Source: three-view drawing plus pictorial views. Frame: mm from the lowest corner of the part. Give positions to 0.01 mm unless a question says otherwise; leave off trailing zeros. Write each loop counter-clockwise with the first axis right and the second up, starting at its lowest first coordinate (ties: lowest second). Pieces come first, ordered by that corner, then holes.
Q1. Pin query (flat end, axial travel): pin 1 (9.5 mm diameter, centred on x = 13, z = 256, fed in from -Y); pin 2 (3 mm diameter, centred on x = 7, y = 86.5, fed in from +Z); pin 3 (3 mm diameter, centred on x = 12.5, y = 304.5, fed in from +Z). Return the tip coordinate at first contact, or that it passes through.
Q2. Cut plane B-B on x = 7.75. Return the cut outline in (y, z).
Q3. Draft query along X for the marked faces 1 and 2. Return one class per face: pulls with the +X half, pulls with the -X half, needs draft (parallel to the pull), parting line crosses it, or undercut.
Q4. Line query: L1, parallel to Y at x = 6, z = 219; L2, parallel to Z at x = 10.25, y = 605.5; L3, parallel to Y at x = 10.25, z = 143. Output: solid intervals per line, ascending.
Q5. Cut plane A-A on z = 32.5. Return the cut outline in (x, y).
Q6. Cut plane D-D on z = 332. Return the cut outline in (x, y).
Q7. Cut plane C-C on y = 545. Return the cut outline in (x, z), plus the area to 3 significant figures.
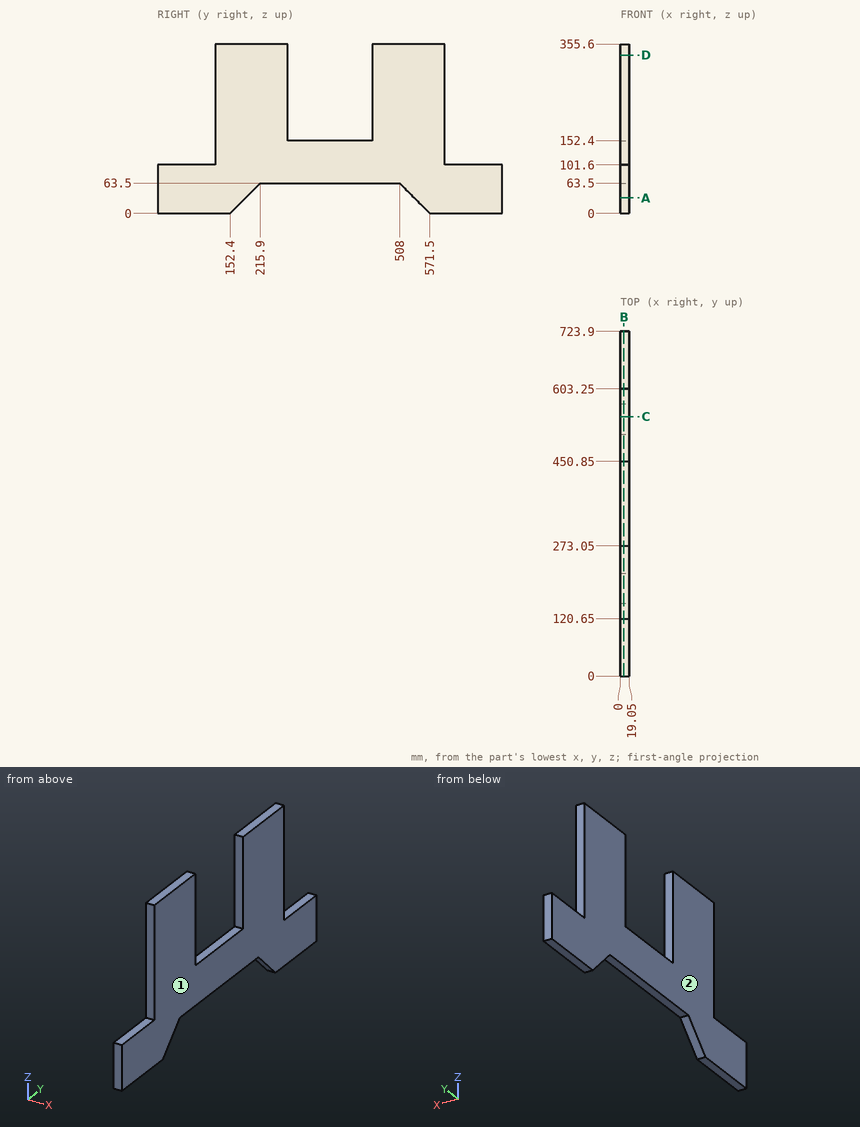
Data:
1. pin 1: stops at y = 120.65
1. pin 2: stops at z = 101.6
1. pin 3: stops at z = 152.4
2. outline: (0, 0) - (152.4, 0) - (215.9, 63.5) - (508, 63.5) - (571.5, 0) - (723.9, 0) - (723.9, 101.6) - (603.25, 101.6) - (603.25, 355.6) - (450.85, 355.6) - (450.85, 152.4) - (273.05, 152.4) - (273.05, 355.6) - (120.65, 355.6) - (120.65, 101.6) - (0, 101.6) - close
3. face 1: pulls with the +X half
3. face 2: pulls with the -X half
4. L1: y = 120.65 to 273.05, 450.85 to 603.25
4. L2: z = 0 to 101.6
4. L3: y = 120.65 to 603.25
5. outline: (0, 0) - (19.05, 0) - (19.05, 184.9) - (0, 184.9) - close; (0, 539) - (19.05, 539) - (19.05, 723.9) - (0, 723.9) - close
6. outline: (0, 120.65) - (19.05, 120.65) - (19.05, 273.05) - (0, 273.05) - close; (0, 450.85) - (19.05, 450.85) - (19.05, 603.25) - (0, 603.25) - close
7. outline: (0, 26.5) - (19.05, 26.5) - (19.05, 355.6) - (0, 355.6) - close
7. area: 6,270 mm2
